For this review, use the dimensioned drawing (mm, ordinates from the lowest corner) and the shaded views. A direction names the side the tool comes from. Coordinates: 2 decimals unless noted, no trailing zeros. Loops run counter-clockwise (first coordinate to the right, second up) from the corner with the lowest first, then second, coordinate; pieces in that order, holes last. Notation, with made-up numbers: (-4, 46) - (1, 46) arc R19 ccw to (1, 74) - close; hole circle Ø1 at (-3.75, 3). An arc over 180 degrees is marked (long way). One line per item, written item: value. Start each with the question number.
1. We need section A-A, the plane y = 7.62. Count the separate pieces of the cut face and the enclosed holes in it, then the cut area to 3 significant figures.
2. Mouldability with a two-part tool opening along X and no side actions: class the marked faces 4, 5 and 6 as +X half, -X half, draft (parallel to the pull), parting line (faces both ways), or undercut.
3. For the marked faces 1, 2 and 3, list the 3-axis set-ups (+Z, -Z, +X, -X, +Y, -Y) from which the entire face can be reached by the end or side of a thin tool; tool diameter is ignored.
4. Insertion check: P1, Ø3.5, axis at x = 33.5, y = 8.5, coming from the +Z side (1 decimal); P2, Ø4.5, axis at x = 33.655, y = 50.419, coming from the -Z side; P3, Ø6, axis at x = 22.5, z = 4.5, coming from the +Y side. Each pin has a flat end and moves straight along its axis. Give the tip position at first contact, or say it passes through.
5. We need section C-C, the plane x = 37. Give the boundary of the cut face in (y, z) (1 decimal).
6. To check wall thickness, follow line 1 (Y direction, x = 6, z = 11.5) (1 decimal); line 2 (Y direction, x = 35.5, z = 3.5); line 3 (X direction, y = 27.5, z = 14). State the ranges of each line that lie inside material, in increasing order.
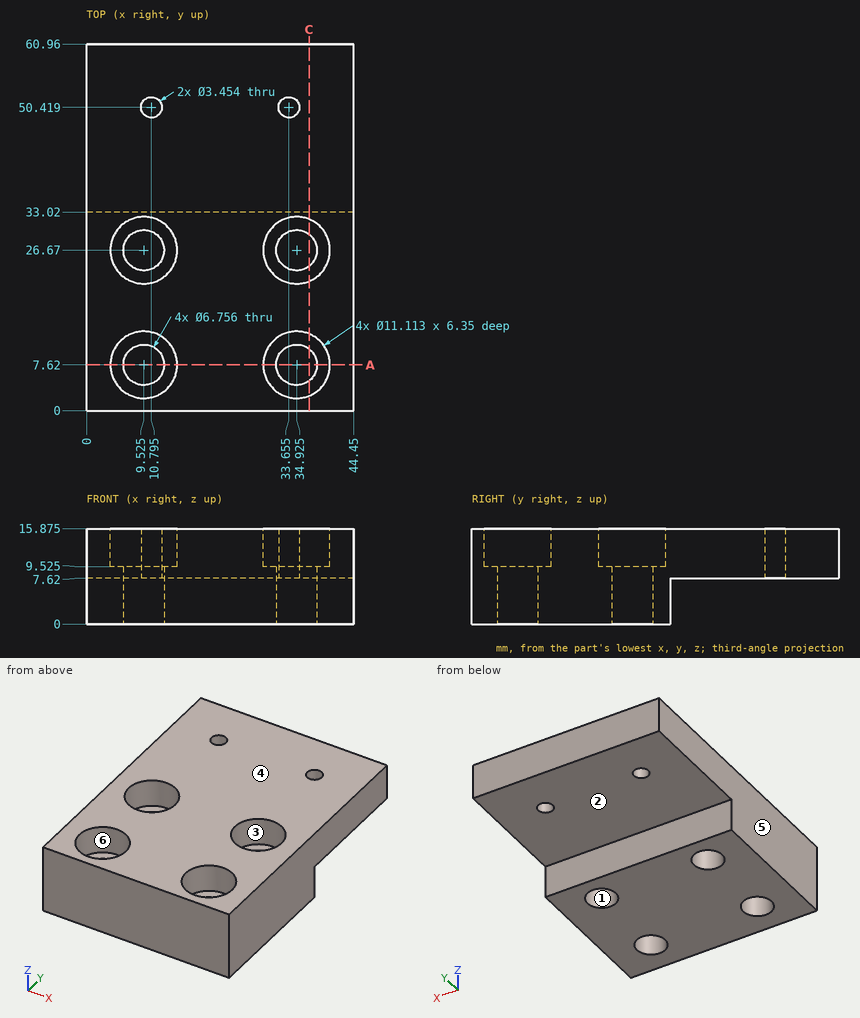
Findings below:
1. separate pieces: 3
1. enclosed holes: 0
1. area: 436 mm2
2. face 4: draft
2. face 5: -X half
2. face 6: undercut
3. face 1: +Z, -Z
3. face 2: -Z, +X, -X, +Y
3. face 3: +Z
4. P1: z = 9.5
4. P2: z = 7.62
4. P3: y = 33.02
5. outline: (0, 0) - (5, 0) - (5, 9.5) - (2.5, 9.5) - (2.5, 15.9) - (0, 15.9) - close; (10.3, 0) - (24, 0) - (24, 9.5) - (21.5, 9.5) - (21.5, 15.9) - (12.8, 15.9) - (12.8, 9.5) - (10.3, 9.5) - close; (29.3, 0) - (33, 0) - (33, 7.6) - (61, 7.6) - (61, 15.9) - (31.8, 15.9) - (31.8, 9.5) - (29.3, 9.5) - close
6. line 1: 0 to 3.3, 11.9 to 22.4, 31 to 61
6. line 2: 0 to 4.29, 10.95 to 23.34, 30 to 33.02
6. line 3: 0 to 4.03, 15.02 to 29.43, 40.42 to 44.45
